Source: CAD feature listing. Evaluate the final solid. Frame: model axes, mm. A direction names the side the tool comes from. Give positions to 0.01 mm unless a question says otherwise; leave off trailing zeros. Order: outer loops, then holes, each group sorted by start corner. A loop starts at its lowest first (then second) coordinate and runs counter-clockwise, first axis right, second up. Notation, with made-up numbers: M 40.25,-8 L 57.25,-8 A20 ccw 57.25,17 Z; hole C 87.25,16 d3. An arc over 180 degrees is marked long. Return JSON: item names as keys, results as strings.
Autodesk Inventor part; units mm, degrees
ref_plane "YZ Plane" through (0, 0, 0) normal (1, 0, 0) x (0, 1, 0)
ref_plane "XZ Plane" through (0, 0, 0) normal (0, 1, 0) x (-1, 0, 0)
ref_plane "XY Plane" through (0, 0, 0) normal (0, 0, 1) x (1, 0, 0)
sketch "草图1" plane through (0, 0, 0) normal (0, 0, 1) x (1, 0, 0)
  arc A0 (10, 0) -> (-10, 0) centre (0, 0) ccw
  line L0 (-15, 0) -> (15, 0)
  line L1 (15, 0) -> (15, -20)
  line L2 (15, -20) -> (-15, -20)
  line L3 (-15, -20) -> (-15, 0)
  circle A1 centre (10, -5) radius 1.5
  circle A2 centre (7, -15) radius 1.5
  circle A3 centre (-10, -5) radius 1.5
  circle A4 centre (-7, -15) radius 1.5
  dimension "d0" = 20
  dimension "d1" = 30
  dimension "d2" = 20
  dimension "d3" = 3
  dimension "d4" = 3
  dimension "d5" = 3
  dimension "d6" = 3
  dimension "d7" = 5
  dimension "d8" = 5
  dimension "d9" = 5
  dimension "d10" = 5
  dimension "d11" = 8
  dimension "d12" = 5
  dimension "d13" = 5
  dimension "d14" = 8
extrude "拉伸1" add sketch "草图1" against normal blind 5
sketch "草图2" plane through (0, 0, -5) normal (0, 0, -1) x (-1, 0, 0)
  circle A0 centre (0, 0) radius 5
  dimension "d17" = 10
extrude "拉伸2" add sketch "草图2" along normal blind 70
chamfer "倒角1" distance 2 angle 45 4 edges at (-11.5, -5, 0) (-8.5, -15, 0) (5.5, -15, 0) (8.5, -5, 0)
properties part number "夹具固定销"
1. First-contact query: pin 1 (2.5 mm diameter, centred on x = -13.5, z = -2, fed in from +Y); pin 2 (5 mm diameter, centred on x = 10, y = -5, fed in from +Z); pin 3 (12 mm diameter, centred on x = 11, y = -7.5, fed in from -Z). Flat tips, straight axial feed; report the tip coordinate or a pass-through.
Evaluation:
{"pin 1": "stops at y = 0", "pin 2": "stops at z = -1", "pin 3": "stops at z = -5"}
2. Section query C-C (y = 3). Return loops of the section in (x, z), then the cut area to 3 significant figures.
Evaluation:
{"outline": "M -9.54,-5 L -4,-5 L -4,-75 L 4,-75 L 4,-5 L 9.54,-5 L 9.54,0 L -9.54,0 Z", "area": "655 mm^2"}
3. Section query A-A (y = -15). Return loops of the section in (x, z), then the cut area to 3 significant figures.
Evaluation:
{"outline": "M -15,-5 L -8.5,-5 L -8.5,-2 L -10.5,0 L -15,0 Z; M -5.5,-5 L 5.5,-5 L 5.5,-2 L 3.5,0 L -3.5,0 L -5.5,-2 Z; M 8.5,-5 L 15,-5 L 15,0 L 10.5,0 L 8.5,-2 Z", "area": "112 mm^2"}
4. Section query B-B (x = 0). Return loops of the section in (y, z), then the cut area to 3 significant figures.
Evaluation:
{"outline": "M -20,-5 L -5,-5 L -5,-75 L 5,-75 L 5,-5 L 10,-5 L 10,0 L -20,0 Z", "area": "850 mm^2"}
5. Section query D-D (z = -23). Return loops of the section in (x, y).
Evaluation:
{"outline": "C 0,0 d10"}
6. Draft query along X for faces 1 (the face through (0, -8, -5)), 2 (the face through (-7.35, -16.59, -1.87)), 3 (the face through (15, -10, -2)). Return one class per face: pulls with the +X half, pulls with the -X half, needs draft (parallel to the pull), parting line crosses it, or undercut.
Evaluation:
{"face 1": "needs draft", "face 2": "undercut", "face 3": "pulls with the +X half"}
7. Ray query, probe 1 along X at (y, z) = (-14.5, -3.5); probe 2 along Z at (x, y) = (5.25, -6.5); probe 3 along Y at (x, z) = (-6.75, -3.5). Return the intervals inside material, ascending.
Evaluation:
{"probe 1": "x = -15 to -8.41, -5.59 to 5.59, 8.41 to 15", "probe 2": "z = -5 to 0", "probe 3": "y = -20 to -16.48, -13.52 to 7.38"}
8. Set-up query: faces 4 (the face through (12, 0, -2)), 5 (the face through (1.08, 4.88, -39.51)), 6 (the face through (-13, 0, -2)). Return all of +Z, -Z, +X, -X, +Y, -Y with unobstructed straight access to the full face (end or side cutting, diameter ignored); none if empty.
Evaluation:
{"face 4": "+Z, -Z, +X, +Y", "face 5": "-Z", "face 6": "+Z, -Z, -X, +Y"}
